CAD build for the part. Positions are in the model's coordinates, mm. A direction names the side the tool comes from. Round coordinates to 2 decimals unless told otherwise and drop trailing zeros. Order: outer loops, then holes, each group sorted by start corner. A loop starts at its lowest first (then second) coordinate and runs counter-clockwise, first axis right, second up. Notation, with made-up numbers: M 8,-13 L 39,-13 A10 cw 39,-7 Z; hole C 19,45.25 d2. An arc over 180 degrees is marked long. Put each result on its own line as item: value.
```python
from build123d import *

# Parameters (mm, degrees)
MODEL_R             = 1.550000002
MODEL_R_2           = 1.550000003
MODEL_R_3           = 1.55
MODEL_W             = 3
MODEL_H             = 10
BOSS_EXTRUDE1_DEPTH = 3


with BuildPart() as part:
    # Model → Boss-Extrude1 (new body)
    with BuildSketch(Plane.XY):
        with BuildLine():
            Line((15.694779571, -8.847330863), (135.394779571, -8.847330863))
            ThreePointArc((135.394779571, -8.847330863), (142.465847383, -5.918398675), (145.394779571, 1.152669137))
            Line((145.394779571, 1.152669137), (145.394779571, 76.099977642))
            ThreePointArc((145.394779571, 76.099977642), (142.435982738, 83.158675114), (135.352544586, 86.057742657))
            Line((135.352544586, 86.057742657), (15.652444586, 86.057742657))
            ThreePointArc((15.652444586, 86.057742657), (8.623648393, 83.128873835), (5.694779571, 76.100077642))
            Line((5.694779571, 76.100077642), (5.694779571, 1.152669137))
            ThreePointArc((5.694779571, 1.152669137), (8.623711759, -5.918398675), (15.694779571, -8.847330863))
        make_face()
        with Locations((81.394879569, 16.599999996)):
            Circle(MODEL_R, mode=Mode.SUBTRACT)
        with Locations((81.394729575, 60.600050002)):
            Circle(MODEL_R, mode=Mode.SUBTRACT)
        with Locations((125.394779569, 16.6)):
            Circle(MODEL_R, mode=Mode.SUBTRACT)
        with Locations((125.394879569, 60.599999996)):
            Circle(MODEL_R, mode=Mode.SUBTRACT)
        with Locations((135.394779571, 76.057742657)):
            Circle(MODEL_R_2, mode=Mode.SUBTRACT)
        with Locations((135.394779571, 1.152669137)):
            Circle(MODEL_R_2, mode=Mode.SUBTRACT)
        with Locations((15.694779571, 76.057742657)):
            Circle(MODEL_R_2, mode=Mode.SUBTRACT)
        with Locations((15.694779571, 1.152669137)):
            Circle(MODEL_R_3, mode=Mode.SUBTRACT)
        with BuildLine():
            Line((101.273453006, 1.866320938), (65.600147072, 37.539741531))
            ThreePointArc((65.600147072, 37.539741531), (65.160808948, 38.600399998), (65.600147072, 39.661058465))
            Line((65.600147072, 39.661058465), (102.334113177, 76.395142639))
            ThreePointArc((102.334113177, 76.395142639), (103.394773848, 76.834484172), (104.455435225, 76.395144343))
            Line((104.455435225, 76.395144343), (140.128859227, 40.721720342))
            ThreePointArc((140.128859227, 40.721720342), (141.007538884, 38.600399998), (140.128859227, 36.479079655))
            Line((140.128859227, 36.479079655), (105.516097102, 1.866317529))
            ThreePointArc((105.516097102, 1.866317529), (103.394774348, 0.987637873), (101.273453006, 1.866320938))
        make_face(mode=Mode.SUBTRACT)
        with Locations((18.315849629, 44.661058465)):
            Rectangle(MODEL_W, MODEL_H, mode=Mode.SUBTRACT)
        with Locations((47.848560539, 43.600399998)):
            Rectangle(MODEL_W, MODEL_H, mode=Mode.SUBTRACT)
    extrude(amount=BOSS_EXTRUDE1_DEPTH)


solid = part.part
```
Item 1: Tool access for faces 4 (the flat face through (49.349, 44, 1)), 5 (the flat face through (75, -8.847, 1)): list every direction of +Z, -Z, +X, -X, +Y, -Y with a clear straight run to the whole face (end or side of a thin tool).
Answers below:
face 4: +Z, -Z
face 5: +Z, -Z, +X, -X, -Y
Item 2: Band-saw the part on B-B on z = 1.95. State how many separate pieces and enclosed holes the cut face has, and give its area (3 significant figures).
Answers below:
separate pieces: 1
enclosed holes: 11
area: 10,000 mm²
Item 3: Probe line 1 along X through (y, z) = (2, 0.9); line 2 along Y through (x, z) = (139, 1.1); line 3 along X through (y, z) = (49, 2.4). List the from-to ranges inside material, lowest first. Write a range as [from, to].
Answers below:
line 1: [5.69, 14.4], [16.99, 101.14], [105.65, 134.1], [136.69, 145.39]
line 2: [-8.17, 35.35], [41.85, 85.39]
line 3: [5.69, 16.82], [19.82, 74.94], [131.85, 145.39]
Item 4: Mould opens along X. For faces 1 (the cylindrical face through (8.701, 83.206, 1.479)), 2 (the flat face through (48, 48.6, 1)), 3 (the flat face through (76, 86.058, 1)) say: pulls with the +X half, pulls with the -X half, needs draft (parallel to the pull), parting line crosses it, or undercut.
Answers below:
face 1: pulls with the -X half
face 2: undercut
face 3: needs draft
Item 5: Pin check, flat tip, straight feed: P1, Ø4, axis at x = 15.69, y = 1.15, coming from the -Z side. Stop position of the tip, or through.
Answers below:
P1: z = 0
Item 6: Band-saw the part on A-A on y = 16.6. Give the cut face in (x, z), and give its area (3 significant figures).
Answers below:
outline: M 5.69,0 L 79.84,0 L 79.84,3 L 5.69,3 Z; M 82.94,0 L 86.54,0 L 86.54,3 L 82.94,3 Z; M 120.25,0 L 123.84,0 L 123.84,3 L 120.25,3 Z; M 126.94,0 L 145.39,0 L 145.39,3 L 126.94,3 Z
area: 299 mm²
